The figure shows three views and two pictorial views of one solid part (mm, origin at its lowest corner). Answer the questions. Coordinates: 2 decimals unless noted, no trailing zeros. Order: outer loops, then holes, each group sorted by start corner. A loop starts at its lowest first (then second) coordinate and runs counter-clockwise, first axis right, second up. Notation, with made-up numbers: (22, 29) -> (32, 29) arc R21 ccw to (32, 50) -> close; hole circle Ø8 at (6.5, 28.25). An arc over 180 degrees is marked (long way). Return JSON: item names as keys, results as strings.
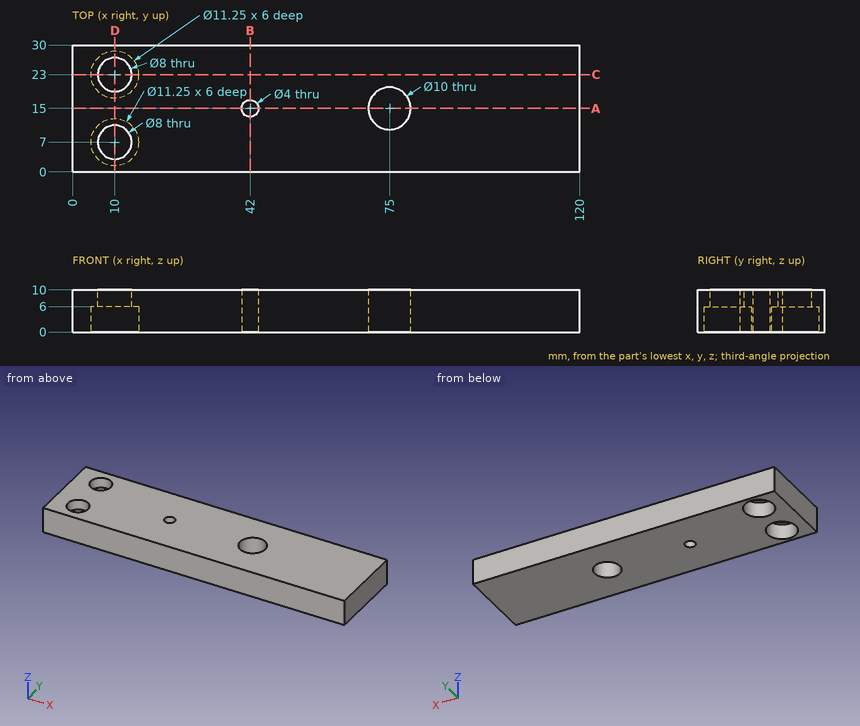
Item 1: Flat-ended cylindrical pins translate along their axes: pin 1 (3.5 mm diameter, centred on x = 7.5, y = 22.5, fed in from -Z); pin 2 (9 mm diameter, centred on x = 75, y = 15, fed in from -Z). Find the tip coordinate at first contact, or state that the pin passes through.
Answer list:
{"pin 1": "z = 6", "pin 2": "through"}
Item 2: The part is cut by section D-D on x = 10. Determine the outline of the cut face in (y, z) (3 decimals), plus the area to 3 significant figures.
Answer list:
{"outline": "(0, 0) -> (1.375, 0) -> (1.375, 6) -> (3, 6) -> (3, 10) -> (0, 10) -> close; (11, 6) -> (12.625, 6) -> (12.625, 0) -> (17.375, 0) -> (17.375, 6) -> (19, 6) -> (19, 10) -> (11, 10) -> close; (27, 6) -> (28.625, 6) -> (28.625, 0) -> (30, 0) -> (30, 10) -> (27, 10) -> close", "area": "101 mm2"}
Item 3: The part is cut by section C-C on y = 23. Determine the outline of the cut face in (x, z) (3 decimals), plus the area to 3 significant figures.
Answer list:
{"outline": "(0, 0) -> (4.375, 0) -> (4.375, 6) -> (6, 6) -> (6, 10) -> (0, 10) -> close; (14, 6) -> (15.625, 6) -> (15.625, 0) -> (120, 0) -> (120, 10) -> (14, 10) -> close", "area": "1,100 mm2"}
Item 4: The part is cut by section A-A on y = 15. Determine the outline of the cut face in (x, z), plus the area to 3 significant figures.
Answer list:
{"outline": "(0, 0) -> (40, 0) -> (40, 10) -> (0, 10) -> close; (44, 0) -> (70, 0) -> (70, 10) -> (44, 10) -> close; (80, 0) -> (120, 0) -> (120, 10) -> (80, 10) -> close", "area": "1,060 mm2"}
Item 5: Find the intervals of material crossed by probe 1 along Y at (x, z) = (10, 4.4) (3 decimals); probe 2 along Y at (x, z) = (10, 7.5); probe 3 along X at (y, z) = (14, 6), in increasing order.
Answer list:
{"probe 1": "0 to 1.375, 12.625 to 17.375, 28.625 to 30", "probe 2": "0 to 3, 11 to 19, 27 to 30", "probe 3": "0 to 40.27, 43.73 to 70.1, 79.9 to 120"}
Item 6: The part is cut by section B-B on x = 42. Determine the outline of the cut face in (y, z).
Answer list:
{"outline": "(0, 0) -> (13, 0) -> (13, 10) -> (0, 10) -> close; (17, 0) -> (30, 0) -> (30, 10) -> (17, 10) -> close"}
